Here's how the part is built. I have some questions about the finished solid (model axes, mm). A direction names the side the tool comes from. Give positions to 0.01 mm unless a question says otherwise; leave off trailing zeros. Loops run counter-clockwise (first coordinate to the right, second up) from the corner with the lowest first, then second, coordinate; pieces in that order, holes last. Notation, with made-up numbers: (-15, 78) - (-6, 78) arc R11 ccw to (-6, 89) - close; hole circle Ø8 at (76.5, -29.75). An arc over 180 degrees is marked (long way). Use a Markdown table: item, result.
from build123d import *

# Parameters (mm, degrees)
SKETCH7_R          = 1.5
SKETCH7_R_2        = 1.7
CUT_EXTRUDE2_DEPTH = 131


with BuildPart() as part:
    # Sketch1 → Revolve1 (revolve)
    with BuildSketch(Plane.XY):
        Polygon((65, -65), (47.5, -82.5), (47.5, -127.679491924), (42.5, -127.679491924), (42.5, -82.5), (60, -65), (60, 0), (65, 0), align=None)
    revolve(axis=Axis((0, 0, 0), (0, -1, 0)))

    # Sketch7 → Cut-Extrude2 (cut, through all)
    with BuildSketch(Plane.XY.offset(-65)):
        with Locations((0, -48.62)):
            Circle(SKETCH7_R)
        with Locations((0, -55.62)):
            Circle(SKETCH7_R)
        with Locations((0, -26.08)):
            Circle(SKETCH7_R_2)
    extrude(amount=CUT_EXTRUDE2_DEPTH, mode=Mode.SUBTRACT)


solid = part.part
(1) If I drill on line 1 (Y direction, x = 0, z = 63.9); line 2 (Y direction, x = 0, z = 61.8); line 3 (Z direction, x = 0, y = -46), over which ranges is the centre line in solid material (lowest first)?
A:
| item | result |
|---|---|
| line 1 | -66.1 to -57.12, -54.12 to -50.12, -47.12 to -27.78, -24.38 to 0 |
| line 2 | -68.2 to -57.12, -54.12 to -50.12, -47.12 to -27.78, -24.38 to 0 |
| line 3 | -65 to -60, 60 to 65 |
(2) Suppose I cut it at A-A on z = 0. Write out the boundary of the cut face in (x, y).
A:
| item | result |
|---|---|
| outline | (-65, -65) - (-47.5, -82.5) - (-47.5, -127.68) - (-42.5, -127.68) - (-42.5, -82.5) - (-60, -65) - (-60, 0) - (-65, 0) - close; (42.5, -127.68) - (47.5, -127.68) - (47.5, -82.5) - (65, -65) - (65, 0) - (60, 0) - (60, -65) - (42.5, -82.5) - close |
(3) We'd pull the mould along Z, two halves only. Please class faces 1 (the face through (-33.727, -104.773, -25.861)), 2 (the face through (-19, 0, -57.5)), 3 (the face through (62, -32.96, 19.52)): pulls with the +Z half, pulls with the -Z half, needs draft (parallel to the pull), parting line crosses it, or undercut.
A:
| item | result |
|---|---|
| face 1 | undercut |
| face 2 | needs draft |
| face 3 | parting line crosses it |
(4) Suppose I cut it at B-B on y = -31. Write out the boundary of the cut face in (x, z).
A:
| item | result |
|---|---|
| outline | circle Ø130 at (0, 0); hole circle Ø120 at (0, 0) |
(5) Will these pins go through, and if not, where does the flat tip stop? pin 1 (2 mm diameter, centred on x = -32.5, y = -112, fed in from -Z); pin 2 (8 mm diameter, centred on x = -48, y = -14.5, fed in from -Z); pin 3 (12 mm diameter, centred on y = -56.5, z = 33, fed in from -X).
A:
| item | result |
|---|---|
| pin 1 | z = -35.55 |
| pin 2 | z = -47.84 |
| pin 3 | x = -59.13 |
(6) On a 3-axis mill with a long thin cutter (end or side, diameter ignored), from which of +Z, -Z, +X, -X, +Y, -Y can I reach the whole of each face in a straight line? I mean faces 4 (the face through (-59.94, -32.04, 2.64)), 5 (the face through (-10.3, -105.41, -46.37)), 6 (the face through (-0.221, -24.394, -62.523)). Say none if no direction works.
A:
| item | result |
|---|---|
| face 4 | +Y |
| face 5 | -Y |
| face 6 | +Z, -Z |
(7) Suppose I cut it at C-C on y = -118. Write out the boundary of the cut face in (x, z), plus the area to 3 significant figures.
A:
| item | result |
|---|---|
| outline | circle Ø95 at (0, 0); hole circle Ø85 at (0, 0) |
| area | 1,410 mm2 |
